Could you check a few things on this model? Use its own coordinates, in mm. Face numbers are marked on the shaded views. Coordinates: 2 decimals unless noted, no trailing zeros. Order: outer loops, then holes, each group sorted by start corner. A loop starts at its lowest first (then second) coordinate and runs counter-clockwise, first axis right, second up. Notation, with made-up numbers: (-25, 0.25) - (15, 0.25) arc R25 ccw to (15, 29.25) - close; hole circle Ø9 at (2, -36). An arc over 180 degrees is marked (long way). Answer as a JSON object with one key per item and string values. Group by question number.
(1) Please list where these lines run through material, in increasing order: probe 1 along Z at (x, y) = (30, -6); probe 2 along X at (y, z) = (-1.25, 89); probe 3 along Z at (x, y) = (29, -2.75).
(2) Imagine slicing it at C-C, the plane y = -2. Write out the boundary of the cut face in (x, z).
(3) Will this pin go through, and if not, where does the flat tip stop? P1, Ø1.5, axis at x = 27.5, y = -2.5, coming from the -Z side.
(4) Imagine slicing it at A-A, the plane z = 86. Write out the boundary of the cut face in (x, y), and give its area (3 significant figures).
(5) We'd pull the mould along Z, two halves only. Please class the marked faces 1, 2, 3 and 4: pulls with the +Z half, pulls with the -Z half, needs draft (parallel to the pull), parting line crosses it, or undercut.
(6) Imagine slicing it at B-B, the plane x = 30. Write out the boundary of the cut face in (y, z).
from build123d import *

# Parameters (mm, degrees)
F0_R     = 8
F1_DEPTH = 10


with BuildPart() as f1:
    # F0 (on Front) → F1 (new body)
    with BuildSketch(Plane.XZ):
        with BuildLine():
            Line((0, 92), (0, 0))
            Line((0, 0), (60, 0))
            Line((60, 0), (60, 92))
            ThreePointArc((60, 92), (57.071068, 99.071068), (50, 102))
            Line((50, 102), (10, 102))
            ThreePointArc((10, 102), (2.928932, 99.071068), (0, 92))
        make_face()
        with Locations((30, 86)):
            Circle(F0_R, mode=Mode.SUBTRACT)
    extrude(amount=F1_DEPTH)


solid = f1.part
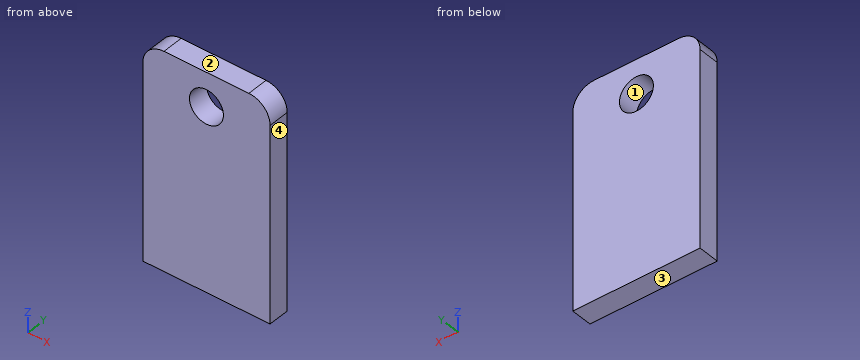
Result set:
{
 "1": {"probe 1": "z = 0 to 78, 94 to 102", "probe 2": "x = 0 to 22.58, 37.42 to 60", "probe 3": "z = 0 to 78.06, 93.94 to 102"},
 "2": {"outline": "(0, 0) - (60, 0) - (60, 92) arc R10 ccw to (50, 102) - (10, 102) arc R10 ccw to (0, 92) - close; hole circle Ø16 at (30, 86)"},
 "3": {"P1": "stops at z = 0"},
 "4": {"outline": "(0, -10) - (22, -10) - (22, 0) - (0, 0) - close; (38, -10) - (60, -10) - (60, 0) - (38, 0) - close", "area": "440 mm^2"},
 "5": {"face 1": "undercut", "face 2": "pulls with the +Z half", "face 3": "pulls with the -Z half", "face 4": "needs draft"},
 "6": {"outline": "(-10, 0) - (0, 0) - (0, 78) - (-10, 78) - close; (-10, 94) - (0, 94) - (0, 102) - (-10, 102) - close"}
}
